```python
from build123d import *

# Parameters (mm, degrees)
SKETCH1_W           = 40
SKETCH1_H           = 50
BOSS_EXTRUDE1_DEPTH = 70
SKETCH2_W           = 30
SKETCH2_H           = 30
CUT_EXTRUDE1_DEPTH  = 51
SKETCH3_W           = 24
SKETCH3_H           = 32
CUT_EXTRUDE2_DEPTH  = 41
SKETCH8_R           = 3.25
CUT_EXTRUDE6_DEPTH  = 41
SKETCH5_R           = 3
CUT_EXTRUDE7_DEPTH  = 36
SKETCH9_W           = 4
SKETCH9_H           = 8
CUT_EXTRUDE8_DEPTH  = 18
CUT_EXTRUDE9_DEPTH  = 51
CHAMFER2_SIZE       = 10
CHAMFER2_SIZE2      = 21.445069205
FILLET3_R           = 40
CHAMFER4_SIZE       = 6
FILLET4_R           = 6


with BuildPart() as part:
    # Sketch1 → Boss-Extrude1 (new body)
    with BuildSketch(Plane(origin=(0, 0, 0), x_dir=(1, 0, 0), z_dir=(0, 1, 0))):
        with Locations((20, 25)):
            Rectangle(SKETCH1_W, SKETCH1_H)
    extrude(amount=BOSS_EXTRUDE1_DEPTH)

    # Sketch2 → Cut-Extrude1 (cut, through all)
    with BuildSketch(Plane.XY):
        with Locations((20, 55)):
            Rectangle(SKETCH2_W, SKETCH2_H)
    extrude(amount=-CUT_EXTRUDE1_DEPTH, mode=Mode.SUBTRACT)

    # Sketch3 → Cut-Extrude2 (cut, through all)
    with BuildSketch(Plane.ZY):
        with Locations((-25, 16)):
            Rectangle(SKETCH3_W, SKETCH3_H)
    extrude(amount=-CUT_EXTRUDE2_DEPTH, mode=Mode.SUBTRACT)

    # Sketch8 → Cut-Extrude6 (cut, through all)
    with BuildSketch(Plane.ZY):
        with Locations((-25, 55)):
            Circle(SKETCH8_R)
    extrude(amount=-CUT_EXTRUDE6_DEPTH, mode=Mode.SUBTRACT)

    # Sketch5 → Cut-Extrude7 (cut)
    with BuildSketch(Plane.ZY):
        with Locations((-43.5, 8.5)):
            Circle(SKETCH5_R)
        with Locations((-6.5, 8.5)):
            Circle(SKETCH5_R)
    extrude(amount=-CUT_EXTRUDE7_DEPTH, mode=Mode.SUBTRACT)

    # Sketch9 → Cut-Extrude8 (cut)
    with BuildSketch(Plane.XZ):
        with Locations((6, -43.5)):
            Rectangle(SKETCH9_W, SKETCH9_H)
        with Locations((6, -6.5)):
            Rectangle(SKETCH9_W, SKETCH9_H)
    extrude(amount=-CUT_EXTRUDE8_DEPTH, mode=Mode.SUBTRACT)

    # Sketch10 → Cut-Extrude9 (cut, through all)
    with BuildSketch(Plane.XY):
        with BuildLine():
            Line((28, 6), (12, 6))
            ThreePointArc((12, 6), (9.5, 8.5), (12, 11))
            Line((12, 11), (28, 11))
            ThreePointArc((28, 11), (30.5, 8.5), (28, 6))
        make_face()
    extrude(amount=-CUT_EXTRUDE9_DEPTH, mode=Mode.SUBTRACT)

    # Chamfer2
    chamfer2_edges = [part.edges().sort_by_distance(p)[0] for p in [
        (0, 32, -25),
    ]]
    chamfer2_side = [part.faces().sort_by_distance(p)[0] for p in [
        (0, 40.838498112, -25),
    ]]
    chamfer(chamfer2_edges, length=CHAMFER2_SIZE, length2=CHAMFER2_SIZE2, reference=chamfer2_side[0])

    # Fillet3
    fillet3_edges = [part.edges().sort_by_distance(p)[0] for p in [
        (21.445069205, 32, -25),
    ]]
    fillet(fillet3_edges, radius=FILLET3_R)

    # Chamfer4
    chamfer4_edges = [part.edges().sort_by_distance(p)[0] for p in [
        (6.704062621, 38.873844259, -13),
        (6.704062621, 38.873844259, -37),
        (21.655271153, 32.948159715, -37),
        (21.655271153, 32.948159715, -13),
        (35.156427855, 32, -37),
        (35.156427855, 32, -13),
    ]]
    chamfer(chamfer4_edges, length=CHAMFER4_SIZE)

    # Fillet4
    fillet4_edges = [part.edges().sort_by_distance(p)[0] for p in [
        (35.156427855, 26, -13),
        (20.35663347, 27.090383672, -13),
        (5.436207835, 32.844787141, -13),
        (6.704062621, 38.873844259, -31),
        (6.704062621, 38.873844259, -19),
        (21.655271153, 32.948159715, -31),
        (21.655271153, 32.948159715, -19),
        (35.156427855, 32, -31),
        (35.156427855, 32, -19),
        (35.156427855, 26, -37),
        (20.35663347, 27.090383672, -37),
        (5.436207835, 32.844787141, -37),
    ]]
    fillet(fillet4_edges, radius=FILLET4_R)


solid = part.part
```
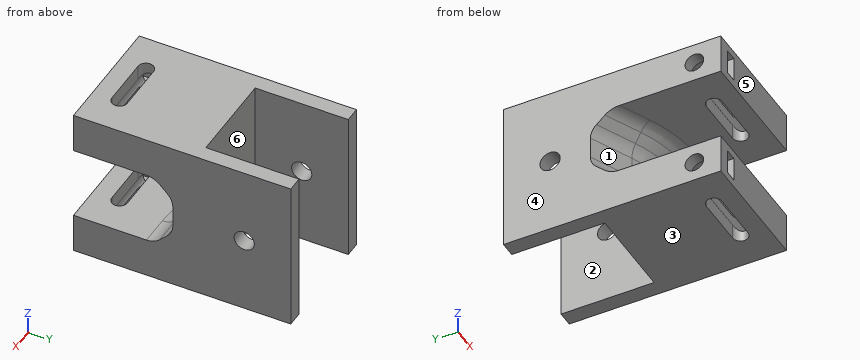
The model under review builds one solid part; all positions refer to its coordinate system, in mm. Face numbers are marked on the shaded views. A direction names the side the tool comes from. Round coordinates to 2 decimals unless told otherwise and drop trailing zeros. Write each loop counter-clockwise with the first axis right and the second up, starting at its lowest first coordinate (ties: lowest second). Pieces come first, ordered by that corner, then holes.
(1) We need section B-B on y = 55. Give the boundary of the cut face in (x, z).
(2) Machinability: for the marked faces 1, 2 and 3, which of the approach directions +Z, -Z, +X, -X, +Y, -Y give a long, thin tool a straight path to every point of the face, cutting with its end or side? Answer none if there is none.
(3) Wall thickness on L1, parallel to Z at x = 9, y = 23; L2, parallel to X at y = 51.5, z = -5.5; L3, parallel to Y at x = 22, z = -12: over which ranges is each line inside the solid? List them lowest first.
(4) Mouldability with a two-part tool opening along X and no side actions: class the marked faces 4, 5 and 6 as +X half, -X half, draft (parallel to the pull), parting line (faces both ways), or undercut.
(5) We need section D-D on z = -43.5. Give the boundary of the cut face in (x, y).
(6) Insertion check: pin 1 (5 mm diameter, centred on x = 23.5, z = -26.5, fed in from +Y). The pin has a flat end and moves straight along its axis. Give the tip position at first contact, or say it passes through.
(7) We need section C-C on y = 20.5. Give the boundary of the cut face in (x, z), and give its area (3 significant figures).
(8) We need section A-A on z = -25. Give the boundary of the cut face in (x, y).
Findings below:
1. outline: (0, -50) - (5, -50) - (5, -28.25) - (0, -28.25) - close; (0, -21.75) - (5, -21.75) - (5, 0) - (0, 0) - close; (35, -50) - (40, -50) - (40, -28.25) - (35, -28.25) - close; (35, -21.75) - (40, -21.75) - (40, 0) - (35, 0) - close
2. face 1: -X, -Y
2. face 2: +Z, -Z, +Y
2. face 3: -Z, +X, -X, +Y, -Y
3. L1: z = -50 to -37, -13 to 0
3. L2: x = 0 to 5, 35 to 40
3. L3: y = 0 to 6, 11 to 40
4. face 4: -X half
4. face 5: draft
4. face 6: undercut
5. outline: (0, 0) - (4, 0) - (4, 5.5) - (0, 5.5) - close; (0, 11.5) - (4, 11.5) - (4, 18) - (8, 18) - (8, 11.5) - (36, 11.5) - (36, 5.5) - (8, 5.5) - (8, 0) - (40, 0) - (40, 70) - (35, 70) - (35, 40) - (5, 40) - (5, 70) - (0, 70) - close
6. pin 1: stops at y = 40
7. outline: (0, -50) - (40, -50) - (40, -37) - (0, -37) - close; (0, -13) - (40, -13) - (40, 0) - (0, 0) - close
7. area: 1,040 mm2
8. outline: (0, 42) - (13.41, 35.75) arc R40 ccw to (30.31, 32) - (40, 32) - (40, 51.75) - (35, 51.75) - (35, 40) - (5, 40) - (5, 51.75) - (0, 51.75) - close; (0, 58.25) - (5, 58.25) - (5, 70) - (0, 70) - close; (35, 58.25) - (40, 58.25) - (40, 70) - (35, 70) - close
